Geometry: final body of the model. Coordinates: model frame, mm. Give positions to 0.01 mm unless a question says otherwise; leave off trailing zeros. Write each loop counter-clockwise with the first axis right and the second up, starting at its lowest first coordinate (ties: lowest second). Pieces come first, ordered by that corner, then holes. Notation, with made-up numbers: (-31, 44) -> (-11, 44) arc R20 cw to (-11, 66) -> close; hole circle Ø10 at (8.5, 82). An arc over 180 degrees is marked (long way). Answer as a JSON object with one key per item and string values. Group by question number.
(1) Contact query for flat-ended pins moving along their axis: pin 1 Ø1.6 at (x, y) = (-3, -7.5) entering from +Z; pin 2 Ø3.5 at (x, z) = (1.5, 18) entering from +Y; pin 3 Ø2.5 at (y, z) = (8, 18.5) entering from -X; pin 4 Ø6 at (x, y) = (14, -9.5) entering from +Z. Output: stop coordinate, or through.
(2) Material intervals for probe 1 along Y at (x, z) = (60.75, 17.55); probe 2 along Z at (x, y) = (36, -0.75); probe 3 along Y at (x, z) = (29.5, 17.5), sorted ascending.
(3) Section query B-B on y = -11. Output: boundary loops of the cut face in (x, z).
(4) Section query A-A on x = 60.75. Output: boundary loops of the cut face in (y, z), plus the area to 3 significant figures.
(5) Section query C-C on x = 20. Output: boundary loops of the cut face in (y, z), plus the area to 3 significant figures.
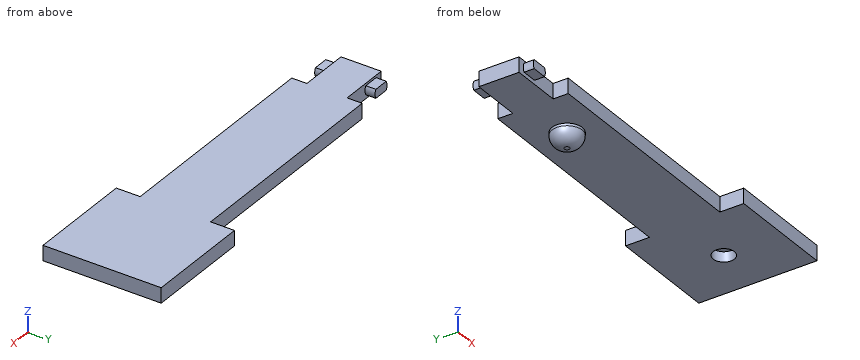
from build123d import *

# Parameters (mm, degrees)
PAD005_DEPTH            = 3
PAD006_DEPTH            = 6
SKETCH006_R             = 2.1
POCKET_DEPTH            = 2
SKETCH007_R             = 3
PAD007_DEPTH            = 3
FILLET001_R             = 2.5
BODY001_ROLL_ANGLE      = 180
BODY001_PLACEMENT_ANGLE = -90


with BuildPart() as part:
    # Sketch005 → Pad005 (new body)
    with BuildSketch(Plane.XY):
        Polygon((-11.75, -33), (11.75, -33), (11.75, -11.5), (7, -11.5), (7, 33), (4, 33), (4, 43), (-4, 43), (-4, 33), (-7, 33), (-7, -11.5), (-11.75, -11.5), align=None)
    extrude(amount=PAD005_DEPTH)

    # Sketch001 → Pad006 (join, symmetric)
    with BuildSketch(Plane.YZ):
        with BuildLine():
            ThreePointArc((41.515544, 0.472742), (41.75, 1.347742), (41.515544, 2.222742))
            Line((41.515544, 2.222742), (38.484456, 2.222742))
            ThreePointArc((38.484456, 2.222742), (38.25, 1.347742), (38.484456, 0.472742))
            Line((41.515544, 0.472742), (38.484456, 0.472742))
        make_face()
    extrude(amount=PAD006_DEPTH, both=True)

    # Sketch006 (on Face5 of Pad006) → Pocket (cut)
    with BuildSketch(Plane.XY.offset(3)):
        with Locations((0, -23)):
            Circle(SKETCH006_R)
    extrude(amount=-POCKET_DEPTH, mode=Mode.SUBTRACT)

    # Sketch007 (on Face5 of Pocket) → Pad007 (join)
    with BuildSketch(Plane.XY.offset(3)):
        with Locations((0, 23)):
            Circle(SKETCH007_R)
    extrude(amount=PAD007_DEPTH)

    # Fillet001
    fillet001_edges = [part.edges().sort_by_distance(p)[0] for p in [
        (-3, 23, 6),
    ]]
    fillet(fillet001_edges, radius=FILLET001_R)


with BuildPart() as part_1:
    # Body001 roll: moved
    add(part.part.rotate(Axis((0, 0, 0), (1, 0, 0)), BODY001_ROLL_ANGLE))


with BuildPart() as part_2:
    # Body001 placement: moved
    add(part_1.part.moved(Location((37.75, -1.865516, 19.218022))).rotate(Axis((37.75, -1.865516, 19.218022), (0, 0, 1)), BODY001_PLACEMENT_ANGLE))


solid = part_2.part
Answer list:
{
 "1": {"pin 1": "z = 18.75", "pin 2": "y = 2.13", "pin 3": "x = 49.25", "pin 4": "z = 19.22"},
 "2": {"probe 1": "-13.62 to -3.97, 0.23 to 9.88", "probe 2": "16.22 to 19.22", "probe 3": "-8.87 to 5.13"},
 "3": {"outline": "(49.25, 16.22) -> (70.75, 16.22) -> (70.75, 19.22) -> (49.25, 19.22) -> close"},
 "4": {"outline": "(-13.62, 16.22) -> (-3.97, 16.22) -> (-3.97, 18.22) -> (0.23, 18.22) -> (0.23, 16.22) -> (9.88, 16.22) -> (9.88, 19.22) -> (-13.62, 19.22) -> close", "area": "62.1 mm2"},
 "5": {"outline": "(-8.87, 16.22) -> (5.13, 16.22) -> (5.13, 19.22) -> (-8.87, 19.22) -> close", "area": "42.0 mm2"}
}
